```python
from build123d import *

# Parameters (mm, degrees)
F0_R     = 16
F1_DEPTH = 635
F2_SIZE  = 2.54
F3_W     = 8
F3_H     = 6
F4_DEPTH = 635.001


with BuildPart() as f1:
    # F0 (on Front) → F1 (new body)
    with BuildSketch(Plane.XZ):
        Circle(F0_R)
    extrude(amount=F1_DEPTH)

    # F2
    f2_edges = [f1.edges().sort_by_distance(p)[0] for p in [
        (-16, 0, 0),
        (-16, -635, 0),
    ]]
    chamfer(f2_edges, length=F2_SIZE)

    # F3 (on face) → F4 (cut, through all)
    with BuildSketch(Plane.XZ.offset(635)):
        with Locations((0, 13.46)):
            Rectangle(F3_W, F3_H)
    extrude(amount=-F4_DEPTH, mode=Mode.SUBTRACT)


solid = f1.part
```
Could you check a few things on this model? Use its own coordinates, in mm. Round coordinates to 2 decimals unless told otherwise and drop trailing zeros. Write each loop counter-clockwise with the first axis right and the second up, starting at its lowest first coordinate (ties: lowest second). Pieces come first, ordered by that corner, then holes.
(1) For pin 1 (2.5 mm diameter, centred on y = -368, z = 13.5, fed in from -X); pin 2 (1 mm diameter, centred on x = 6, y = -125, fed in from -Z) (3 decimals); pin 3 (5.5 mm diameter, centred on y = -226.5, z = 12, fed in from +X), each with a flat end and sliding along its axis, tell me the tip position at first contact or that it passes through.
Findings below:
pin 1: stops at x = -10.29
pin 2: stops at z = -15.025
pin 3: stops at x = 13.06
(2) If I drill on probe 1 along X at (y, z) = (-198, 1.5); probe 2 along X at (y, z) = (-510.5, 12); probe 3 along X at (y, z) = (-399.5, -0.5), over which ranges is the centre line in solid material (lowest first)?
Findings below:
probe 1: x = -15.93 to 15.93
probe 2: x = -10.58 to -4, 4 to 10.58
probe 3: x = -15.99 to 15.99
(3) Suppose I cut it at A-A on y = -397.5. Write out the boundary of the cut face in (x, z), and give its area (3 significant figures).
Findings below:
outline: (-4, 10.46) - (-4, 15.49) arc R16 ccw (long way) to (4, 15.49) - (4, 10.46) - close
area: 761 mm2
